Design review of the part built by this model. Coordinates are the model's own, in mm. A direction names the side the tool comes from. Round coordinates to 2 decimals unless told otherwise and drop trailing zeros. Loops run counter-clockwise (first coordinate to the right, second up) from the corner with the lowest first, then second, coordinate; pieces in that order, holes last. Notation, with made-up numbers: M 36,65 L 54,65 A23 ccw 54,88 Z; hole C 64.25,-14 d3. An arc over 180 degrees is marked long. Use a Markdown table: item, result.
from build123d import *

# Parameters (mm, degrees)
F0_R     = 2.5
F1_DEPTH = 15
F2_R     = 5
F4_DEPTH = 5
F5_DEPTH = 2.5


with BuildPart() as f1:
    # F0 (on Front) → F1 (new body)
    with BuildSketch(Plane.XZ):
        with BuildLine():
            Line((-20.85, 20.85), (-20.85, 0))
            Line((-20.85, 0), (-20.85, -20.85))
            Line((-20.85, -20.85), (0, -20.85))
            Line((0, -20.85), (20.85, -20.85))
            Line((20.85, -20.85), (20.85, 0))
            Line((20.85, 0), (20.85, 20.85))
            Line((20.85, 20.85), (10.425, 20.85))
            Line((10.425, 20.85), (10.425, 47.277337854))
            ThreePointArc((10.425, 47.277337854), (24.8578784585, 67.3380686447), (15, 90))
            Line((15, 90), (15, 110))
            Line((15, 110), (5, 110))
            Line((5, 110), (5, 84.1421356237))
            ThreePointArc((5, 84.1421356237), (14.9999953406, 69.9881770745), (4.9777002722, 55.85))
            Line((4.9777002722, 55.85), (-10.425, 55.85))
            Line((-10.425, 55.85), (-10.425, 20.85))
            Line((-10.425, 20.85), (-20.85, 20.85))
        make_face()
        Polygon((-12.85, 12.85), (0, 12.85), (12.85, 12.85), (12.85, 0), (12.85, -12.85), (0, -12.85), (-12.85, -12.85), (-12.85, 0), align=None, mode=Mode.SUBTRACT)
        with Locations((-5.425, 50.85)):
            Circle(F0_R, mode=Mode.SUBTRACT)
    extrude(amount=F1_DEPTH)

    # F2
    f2_edges = [f1.edges().sort_by_distance(p)[0] for p in [
        (-10.425, -7.5, 55.85),
    ]]
    fillet(f2_edges, radius=F2_R)

    # F3 (on face) → F4 (cut)
    with BuildSketch(Plane.XZ.offset(15)):
        with BuildLine():
            Line((-0.425, 55.85), (-5.425, 55.85))
            ThreePointArc((-5.425, 55.85), (-8.9605339059, 54.3855339059), (-10.425, 50.85))
            Line((-10.425, 50.85), (-10.425, 45.85))
            Line((-10.425, 45.85), (-5.425, 45.85))
            ThreePointArc((-5.425, 45.85), (-1.8894660941, 47.3144660941), (-0.425, 50.85))
            Line((-0.425, 50.85), (-0.425, 55.85))
        make_face()
    extrude(amount=-F4_DEPTH, mode=Mode.SUBTRACT)

    # F5 (add): a face of the model
    f5_faces = [f1.faces().sort_by_distance(p)[0] for p in [
        (4.1569852553, -15, 31.7276341026),
    ]]
    extrude(f5_faces, amount=F5_DEPTH)


solid = f1.part
1. Take a section at A-A on x = 1. Give the boundary of the cut face in (y, z), and give its area (4 significant figures).
Check values:
| item | result |
|---|---|
| outline | M -17.5,-20.85 L 0,-20.85 L 0,-12.85 L -17.5,-12.85 Z; M -17.5,12.85 L 0,12.85 L 0,55.85 L -17.5,55.85 Z |
| area | 892.5 mm² |
2. Machinability: for faces 1 (the face through (-12.85, -9, 0)), 2 (the face through (-1.929, -13.698, 47.276)), 3 (the face through (20.85, -9, 0)), 4 (the face through (1, -7, 55.85)), which of the approach directions +Z, -Z, +X, -X, +Y, -Y give a long, thin tool a straight path to every point of the face, cutting with its end or side? Answer none if there is none.
Check values:
| item | result |
|---|---|
| face 1 | +Y, -Y |
| face 2 | +Z, -X, -Y |
| face 3 | -Z, +X, +Y, -Y |
| face 4 | +Z, -X, +Y, -Y |
3. Insertion check: pin 1 (10 mm diameter, centred on y = -15, z = 62.5, fed in from +X); pin 2 (1.5 mm diameter, centred on y = -13, z = 54, fed in from -X) (3 decimals); pin 3 (5 mm diameter, centred on y = -7, z = 99.5, fed in from +X); pin 4 (4.5 mm diameter, centred on x = -5.425, z = 50.85, fed in from +Y). Each pin has a flat end and moves straight along its axis. Give the tip position at first contact, or say it passes through.
Check values:
| item | result |
|---|---|
| pin 1 | stops at x = 24.87 |
| pin 2 | stops at x = -0.425 |
| pin 3 | stops at x = 15 |
| pin 4 | passes through |
4. Wall thickness on line 1 along Z through (x, y) = (-7.5, -10.5); line 2 along X through (y, z) = (-15.75, -11): over which ranges is each line inside the solid? List them lowest first. Write a range as from..to.
Check values:
| item | result |
|---|---|
| line 1 | z = -20.85..-12.85, 12.85..45.85 |
| line 2 | x = -20.85..-12.85, 12.85..20.85 |
5. The part is to be moulded in two halves that separate along Z. For faces 5 (the face through (10, -9, 110)), 6 (the face through (-5.97, -4.93, 48.41)), 7 (the face through (-8, -10, 50)), say which applies: pulls with the +Z half, pulls with the -Z half, needs draft (parallel to the pull), parting line crosses it, or undercut.
Check values:
| item | result |
|---|---|
| face 5 | pulls with the +Z half |
| face 6 | undercut |
| face 7 | needs draft |
6. Take a section at B-B on y = -4.5. Give the boundary of the cut face in (x, z) (3 decimals), and give its area (3 significant figures).
Check values:
| item | result |
|---|---|
| outline | M -20.85,-20.85 L 20.85,-20.85 L 20.85,20.85 L 10.425,20.85 L 10.425,47.277 A25 ccw 15,90 L 15,110 L 5,110 L 5,84.142 A15 cw 4.978,55.85 L -5.425,55.85 A5 ccw -10.425,50.85 L -10.425,20.85 L -20.85,20.85 Z; hole M -12.85,-12.85 L 12.85,-12.85 L 12.85,12.85 L -12.85,12.85 Z; hole C -5.425,50.85 d5 |
| area | 2,430 mm² |
7. Take a section at C-C on x = -18. Give the boundary of the cut face in (y, z), and give its area (3 significant figures).
Check values:
| item | result |
|---|---|
| outline | M -17.5,-20.85 L 0,-20.85 L 0,20.85 L -17.5,20.85 Z |
| area | 730 mm² |
